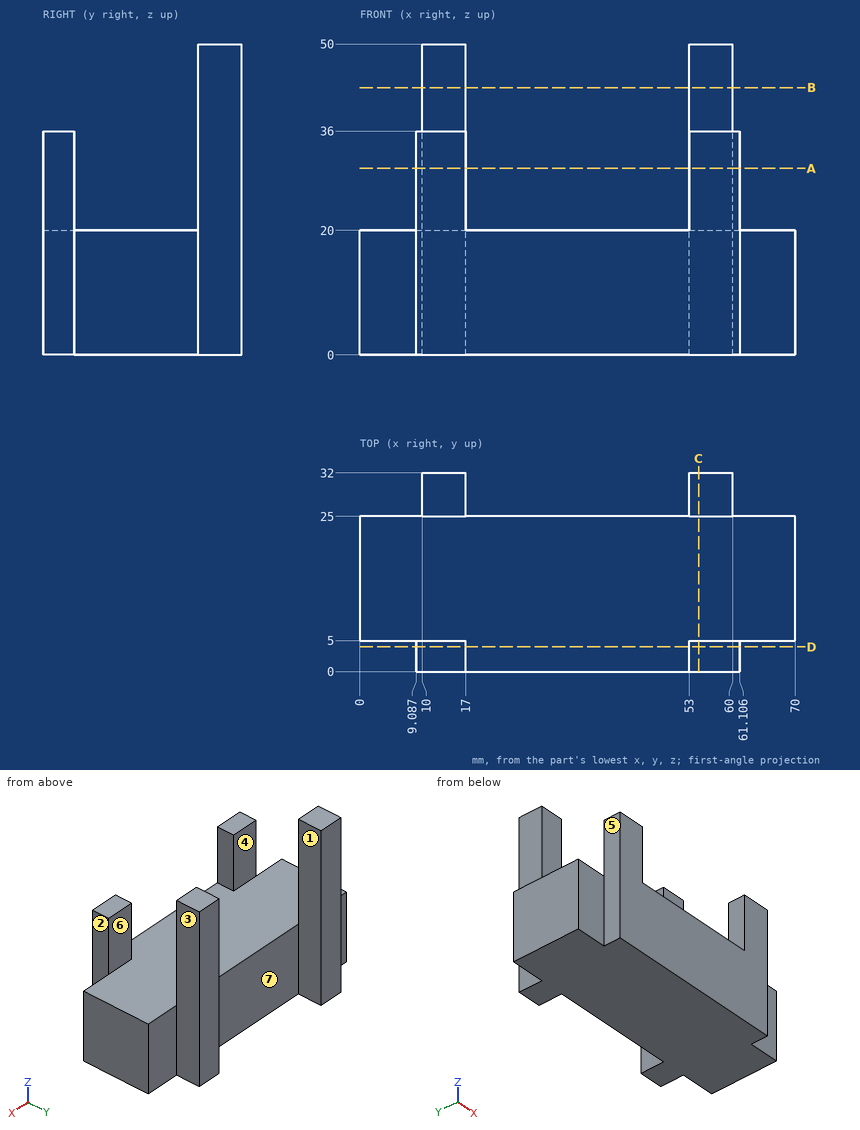
Could you check a few things on this drawing? It's one solid part, dimensions in mm from its lowest x, y, z. A direction names the side the tool comes from. Give positions to 0.01 mm unless a question says otherwise; leave off trailing zeros. Write each loop counter-clockwise with the first axis right and the second up, starting at its lowest first coordinate (ties: lowest second). Pieces come first, ordered by that corner, then holes.
(1) Imagine slicing it at D-D, the plane y = 4. Write out the boundary of the cut face in (x, z) (1 decimal).
Output values:
outline: (9.1, 0) - (61.1, 0) - (61.1, 36) - (53, 36) - (53, 20) - (17, 20) - (17, 36) - (9.1, 36) - close
(2) Imagine slicing it at A-A, the plane z = 30. Write out the boundary of the cut face in (x, y) (1 decimal).
Output values:
outline: (9.1, 0) - (17, 0) - (17, 5) - (9.1, 5) - close; (10, 25) - (17, 25) - (17, 32) - (10, 32) - close; (53, 0) - (61.1, 0) - (61.1, 5) - (53, 5) - close; (53, 25) - (60, 25) - (60, 32) - (53, 32) - close
(3) Thinking about a two-plate mould opening in Y: for the marked faces 4, 5, 6 and 7, which applies, pulls with the +Y half, pulls with the -Y half, needs draft (parallel to the pull), parting line crosses it, or undercut?
Output values:
face 4: undercut
face 5: needs draft
face 6: undercut
face 7: pulls with the +Y half
(4) Imagine slicing it at B-B, the plane z = 43. Write out the boundary of the cut face in (x, y).
Output values:
outline: (10, 25) - (17, 25) - (17, 32) - (10, 32) - close; (53, 25) - (60, 25) - (60, 32) - (53, 32) - close
(5) Will these pins go through, and if not, where does the flat tip stop? pin 1 (5.5 mm diameter, centred on y = 3, z = 29, fed in from -X); pin 2 (1.5 mm diameter, centred on x = 12.5, y = 2, fed in from +Z); pin 3 (8 mm diameter, centred on x = 4, z = 15, fed in from +Y).
Output values:
pin 1: stops at x = 9.09
pin 2: stops at z = 36
pin 3: stops at y = 25
(6) If I drill on L1, parallel to X at y = 27, z = 27.5; L2, parallel to Y at x = 11, z = 36.5; L3, parallel to X at y = 2.5, z = 32 (1 decimal), over which ranges is the centre line in solid material (lowest first)?
Output values:
L1: x = 10 to 17, 53 to 60
L2: y = 25 to 32
L3: x = 9.1 to 17, 53 to 61.1
(7) On a 3-axis mill with a long thin cutter (end or side, diameter ignored), from which of +Z, -Z, +X, -X, +Y, -Y can I reach the whole of each face in a straight line? I mean the marked faces 1, 2 and 3. Say none if no direction works.
Output values:
face 1: +Z, -Z, +Y
face 2: +Z, -Z, +X, -Y
face 3: +Z, -Z, +X, +Y
(8) Imagine slicing it at C-C, the plane x = 54.5. Write out the boundary of the cut face in (y, z).
Output values:
outline: (0, 0) - (32, 0) - (32, 50) - (25, 50) - (25, 20) - (5, 20) - (5, 36) - (0, 36) - close
